from build123d import *

# Parameters (mm, degrees)
F0_R     = 10
F1_DEPTH = 19
F2_R     = 15
F3_DEPTH = 30
F4_R     = 25
F5_DEPTH = 10
F6_R     = 15
F7_DEPTH = 20
F9_DEPTH = 19


with BuildPart() as f1:
    # F0 (on Right) → F1 (new body)
    with BuildSketch(Plane.YZ):
        Circle(F0_R)
    extrude(amount=F1_DEPTH)

    # F2 (on face) → F3 (join)
    with BuildSketch(Plane.YZ.offset(19)):
        Circle(F2_R)
    extrude(amount=F3_DEPTH)

    # F4 (on face) → F5 (join)
    with BuildSketch(Plane.YZ.offset(49)):
        Circle(F4_R)
    extrude(amount=F5_DEPTH)

    # F6 (on face) → F7 (join)
    with BuildSketch(Plane.YZ.offset(59)):
        Circle(F6_R)
    extrude(amount=F7_DEPTH)

    # F8 (on face) → F9 (cut, through all)
    with BuildSketch(Plane(origin=(0, 0, 0), x_dir=(0, -1, 0), z_dir=(-1, 0, 0))):
        with BuildLine():
            ThreePointArc((6, 8), (0, 10), (-6, 8))
            Line((-6, 8), (6, 8))
        make_face()
    extrude(amount=-F9_DEPTH, mode=Mode.SUBTRACT)

    # F10: F1 across face


with BuildPart() as f1_1:
    add(f1.part)
    add(f1.part.mirror(Plane.YZ.offset(79)))


solid = f1_1.part
The model under review builds one solid part; all positions refer to its coordinate system, in mm. A direction names the side the tool comes from. Round coordinates to 2 decimals unless told otherwise and drop trailing zeros. Loops run counter-clockwise (first coordinate to the right, second up) from the corner with the lowest first, then second, coordinate; pieces in that order, holes last. Notation, with made-up numbers: (-16, 44) -> (19, 44) arc R17 cw to (19, 51) -> close; hole circle Ø7 at (49, 3.5). An arc over 180 degrees is marked (long way). Return JSON: item names as keys, results as strings.
(1) The part is to be moulded in two halves that separate along X. For faces 5 (the flat face through (99, 11, -11)), 6 (the flat face through (9, 0, 8)), 7 (the flat face through (158, 0, -1)), say which applies: released by +X, released by -X, zero draft, split by the parting line, or undercut.
Solved:
{"face 5": "undercut", "face 6": "zero draft", "face 7": "released by +X"}
(2) For line 1 (X direction, y = 12, z = -10); line 2 (X direction, y = -2, z = 9); line 3 (Z direction, x = 26, y = 0.5), list the stretches that pass through material, from the lowest coordinate up.
Solved:
{"line 1": "49 to 59, 99 to 109", "line 2": "19 to 139", "line 3": "-14.99 to 14.99"}
(3) Add section A-A on y = 0. Write out the cut boundary in (x, z), plus the area to 3 significant figures.
Solved:
{"outline": "(0, -10) -> (19, -10) -> (19, -15) -> (49, -15) -> (49, -25) -> (59, -25) -> (59, -15) -> (99, -15) -> (99, -25) -> (109, -25) -> (109, -15) -> (139, -15) -> (139, -10) -> (158, -10) -> (158, 8) -> (139, 8) -> (139, 15) -> (109, 15) -> (109, 25) -> (99, 25) -> (99, 15) -> (59, 15) -> (59, 25) -> (49, 25) -> (49, 15) -> (19, 15) -> (19, 8) -> (0, 8) -> close", "area": "4,680 mm2"}
(4) Add section C-C on x = 35.5. Write out the cut boundary in (y, z).
Solved:
{"outline": "circle Ø30 at (0, 0)"}
(5) For pin 1 (1.5 mm diameter, centred on y = 0, z = 1, fed in from -X); pin 2 (10 mm diameter, centred on x = 17.5, z = 11, fed in from +Y); pin 3 (3.5 mm diameter, centred on x = 148.5, y = 2.5, fed in from +Z); pin 4 (3 mm diameter, centred on x = 38.5, z = 1, fed in from +Y), all flat-tipped, find the tip position at first contact; note any pin that passes through.
Solved:
{"pin 1": "x = 0", "pin 2": "y = 13.64", "pin 3": "z = 8", "pin 4": "y = 15"}
(6) Add section B-B on z = 0. Write out the cut boundary in (x, y).
Solved:
{"outline": "(0, -10) -> (19, -10) -> (19, -15) -> (49, -15) -> (49, -25) -> (59, -25) -> (59, -15) -> (99, -15) -> (99, -25) -> (109, -25) -> (109, -15) -> (139, -15) -> (139, -10) -> (158, -10) -> (158, 10) -> (139, 10) -> (139, 15) -> (109, 15) -> (109, 25) -> (99, 25) -> (99, 15) -> (59, 15) -> (59, 25) -> (49, 25) -> (49, 15) -> (19, 15) -> (19, 10) -> (0, 10) -> close"}
(7) Add section D-D on y = -13.5. Write out the cut boundary in (x, z).
Solved:
{"outline": "(19, -6.54) -> (49, -6.54) -> (49, -21.04) -> (59, -21.04) -> (59, -6.54) -> (99, -6.54) -> (99, -21.04) -> (109, -21.04) -> (109, -6.54) -> (139, -6.54) -> (139, 6.54) -> (109, 6.54) -> (109, 21.04) -> (99, 21.04) -> (99, 6.54) -> (59, 6.54) -> (59, 21.04) -> (49, 21.04) -> (49, 6.54) -> (19, 6.54) -> close"}
(8) For faces 1 (the flat face through (149, 0, 8)), 2 (the flat face through (139, 3, -10)), 3 (the flat face through (19, 3, -10)), 4 (the flat face through (59, 11, -11)), list the 3-axis set-ups (+Z, -Z, +X, -X, +Y, -Y) from which the entire face can be reached by the end or side of a thin tool; tool diameter is ignored.
Solved:
{"face 1": "+Z, +X, +Y, -Y", "face 2": "+X", "face 3": "-X", "face 4": "none"}
